Autodesk Inventor part; units mm, degrees
ref_plane "YZ Plane" through (0, 0, 0) normal (1, 0, 0) x (0, 1, 0)
ref_plane "XZ Plane" through (0, 0, 0) normal (0, 1, 0) x (-1, 0, 0)
ref_plane "XY Plane" through (0, 0, 0) normal (0, 0, 1) x (1, 0, 0)
sketch "Outer Diameter Sketch" plane through (0, 0, 0) normal (0, 1, 0) x (-1, 0, 0)
  line L0 (0, -28.0163) -> (0, 28.3344) construction
  line L1 (17.1062, 0) -> (-23.8822, 0) construction
  line L2 (3.4641, -6) -> (6.9282, 0)
  line L3 (6.9282, 0) -> (3.4641, 6)
  line L4 (3.4641, 6) -> (-3.4641, 6)
  line L5 (-3.4641, 6) -> (-6.9282, 0)
  line L6 (-6.9282, 0) -> (-3.4641, -6)
  line L7 (-3.4641, -6) -> (3.4641, -6)
  line L8 (0, -6) -> (0, 6) construction
  line L9 (-6.9282, 0) -> (6.9282, 0) construction
  point P0 (0, 0)
  dimension "d23" = 120
  dimension "d25" = 120
  dimension "d27" = 120
  dimension "d29" = 120
  dimension "d31" = 120
  dimension "d32" = 12
extrude "Outer Diameter Extrusion" add sketch "Outer Diameter Sketch" along normal mid plane 130
sketch "Sketch2" plane through (0, 0, 0) normal (1, 0, 0) x (0, 1, 0)
  circle A0 centre (-7, 0) radius 4.5
  line L0 (-72, 0) -> (-7, 0) construction
  line L1 (-7, 0) -> (58, 0) construction
  circle A1 centre (7, 0) radius 4.5
  circle A2 centre (21, 0) radius 4.5
  circle A3 centre (35, 0) radius 4.5
  circle A4 centre (-21, 0) radius 4.5
  circle A5 centre (-7, 0) radius 4.5
  circle A6 centre (7, 0) radius 4.5
  circle A7 centre (21, 0) radius 4.5
  circle A8 centre (-35, 0) radius 4.5
  circle A9 centre (-21, 0) radius 4.5
  circle A10 centre (-7, 0) radius 4.5
  circle A11 centre (7, 0) radius 4.5
  circle A12 centre (-49, 0) radius 4.5
  circle A13 centre (-35, 0) radius 4.5
  circle A14 centre (-21, 0) radius 4.5
  circle A15 centre (-7, 0) radius 4.5
  line L2 (0, 54.0285) -> (0, -72.3739) construction
  circle A16 centre (49, 0) radius 4.5
  circle A17 centre (35, 0) radius 4.5
  circle A18 centre (21, 0) radius 4.5
  circle A19 centre (7, 0) radius 4.5
  dimension "d3" = 9
  dimension "d5" = 130
  dimension "d8" = 14
  dimension "d11" = 14
  dimension "d47" = 7
  dimension "d48" = 7
extrude "Peg Extrusions" add sketch "Sketch2" along normal mid plane 32
sketch "Sketch3" plane through (0, -65, 0) normal (0, -1, 0) x (1, 0, 0)
  line L0 (1.55, -2.6847) -> (-1.55, -2.6847)
  line L1 (-1.55, -2.6847) -> (-3.1, 0)
  line L2 (-3.1, 0) -> (-1.55, 2.6847)
  line L3 (-1.55, 2.6847) -> (1.55, 2.6847)
  line L4 (1.55, 2.6847) -> (3.1, 0)
  line L5 (3.1, 0) -> (1.55, -2.6847)
  line L6 (3.1, 0) -> (-3.1, 0) construction
  line L7 (0, 2.6847) -> (0, -2.6847) construction
  line L8 (10.3659, 0) -> (-11.745, 0) construction
  line L9 (0, -9.4896) -> (0, 9.303) construction
  point P0 (0, 0)
  dimension "d33" = 3.1
  dimension "d34" = 3.1
  dimension "d35" = 120
  dimension "d36" = 3.1
  dimension "d37" = 120
  dimension "d38" = 3.1
  dimension "d39" = 120
  dimension "d40" = 3.1
  dimension "d41" = 120
extrude "Inner Hex Cut" cut sketch "Sketch3" against normal up to surface (130 mm away)
equation "\"d1\" = outL"
equation "\"d3\" = pegD"
equation "\"d5\" = outL"
equation "\"d47\" = 0.5 * d8"
equation "\"d14\" = pegL + 2 * outD"
equation "\"d33\" = inhexSL"
equation "\"d34\" = inhexSL"
equation "\"d36\" = inhexSL"
equation "\"d38\" = inhexSL"
equation "\"d40\" = inhexSL"
equation "\"d42\" = pegL + 2 * outD"
equation "\"outD\" = 12"
equation "\"inhexSL\" = 3.1"
equation "\"outL\" = 130"
equation "\"pegL\" = 8"
equation "\"pegD\" = 9"
equation "\"outhexSL\" = 5"
properties part number "Peg Spinner V3"
Can you work these out from the model? Positions are in its coordinate system, mm. A direction names the side the tool comes from. Give positions to 0.01 mm unless a question says otherwise; leave off trailing zeros. Write each loop counter-clockwise with the first axis right and the second up, starting at its lowest first coordinate (ties: lowest second). Pieces come first, ordered by that corner, then holes. Notation, with made-up numbers: M -21.5,84.25 L -1.5,84.25 A21 cw -1.5,122.25 Z; hole C 38,71 d10. An arc over 180 degrees is marked long. Answer in a Markdown table with one row per item. Add a question column.
Item 1: Imagine slicing it at A-A, the plane y = 35. Write out the boundary of the cut face in (x, z).
Item 2: Imagine slicing it at B-B, the plane y = -24. Write out the boundary of the cut face in (x, z), plus the area to 3 significant figures.
Item 3: We'd pull the mould along Y, two halves only. Please class faces 4 (the flat face through (-16, 21, 0)), 5 (the cylindrical face through (10.079, 53.292, -1.352)), 6 (the flat face through (0, -65, 3)), 7 (the flat face through (5.22, -0.91, -2.96)): released by +Y, released by -Y, zero draft, split by the parting line, or undercut.
Item 4: On a 3-axis mill with a long thin cutter (end or side, diameter ignored), from which of +Z, -Z, +X, -X, +Y, -Y can I reach the whole of each face in a straight line? I mean faces 1 (the flat face through (0, -1, -2.685)), 2 (the cylindrical face through (-10.079, 39.292, 1.352)), 3 (the cylindrical face through (10.079, 11.292, -1.352)). Say none if no direction works.
Item 5: For pin 1 Ø5 at (y, z) = (-16, 1) entering from -X; pin 2 Ø4 at (y, z) = (28.5, -3) entering from -X; pin 3 Ø1.5 at (x, y) = (10, -31) entering from +Z; pin 4 Ø12 at (x, y) = (12.5, 36) entering from -Z, each with a flat end and sliding along its axis, tell me the tip position at first contact or that it passes through.
Item 6: Please list where these lines run through material, in increasing order: L1, parallel to Z at x = 1.5, y = 45.5; L2, parallel to X at y = -8.5, z = -0.75; L3, parallel to Z at x = -2.5, y = 49.
Evaluation:
| question | item | result |
|---|---|---|
| 1 | outline | M -16,-4.5 L -4.33,-4.5 L -3.46,-6 L 3.46,-6 L 4.33,-4.5 L 16,-4.5 L 16,4.5 L 4.33,4.5 L 3.46,6 L -3.46,6 L -4.33,4.5 L -16,4.5 Z; hole M -3.1,0 L -1.55,-2.68 L 1.55,-2.68 L 3.1,0 L 1.55,2.68 L -1.55,2.68 Z |
| 2 | outline | M -16,-3.35 L -4.99,-3.35 L -3.46,-6 L 3.46,-6 L 4.99,-3.35 L 16,-3.35 L 16,3.35 L 4.99,3.35 L 3.46,6 L -3.46,6 L -4.99,3.35 L -16,3.35 Z; hole M -3.1,0 L -1.55,-2.68 L 1.55,-2.68 L 3.1,0 L 1.55,2.68 L -1.55,2.68 Z |
| 2 | area | 234 mm² |
| 3 | face 4 | zero draft |
| 3 | face 5 | undercut |
| 3 | face 6 | released by -Y |
| 3 | face 7 | undercut |
| 4 | face 1 | +Y, -Y |
| 4 | face 2 | -X |
| 4 | face 3 | +X |
| 5 | pin 1 | stops at x = -16 |
| 5 | pin 2 | stops at x = -6.35 |
| 5 | pin 3 | stops at z = 3.11 |
| 5 | pin 4 | stops at z = -4.5 |
| 6 | L1 | z = -6 to -2.68, 2.68 to 6 |
| 6 | L2 | x = -16 to -2.67, 2.67 to 16 |
| 6 | L3 | z = -6 to -1.04, 1.04 to 6 |
